The model under review builds one solid part; all positions refer to its coordinate system, in mm. Face numbers are marked on the shaded views. A direction names the side the tool comes from. Round coordinates to 2 decimals unless told otherwise and drop trailing zeros. Write each loop counter-clockwise with the first axis right and the second up, starting at its lowest first coordinate (ties: lowest second). Pieces come first, ordered by that corner, then holes. Notation, with made-up numbers: (55.25, 57.5) - (62.25, 57.5) arc R18 cw to (62.25, 91.5) - close; hole circle Ø7 at (-37, 60.25). An arc over 180 degrees is marked (long way). Return JSON: item names as keys, results as strings.
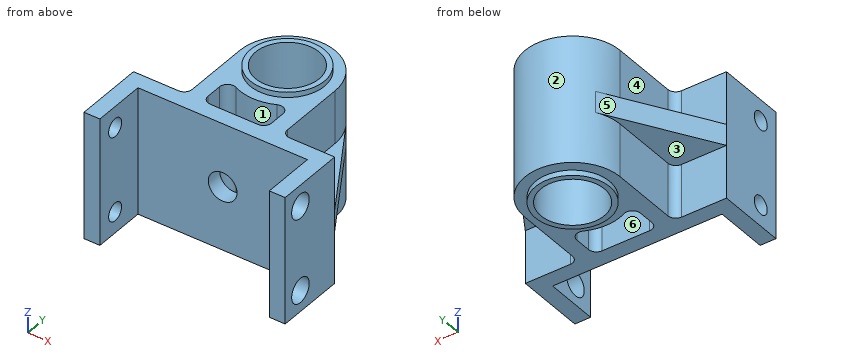
from build123d import *

# Parameters (mm, degrees)
F0_R           = 4.7625
F1_DEPTH       = 19.05
F2_R           = 1.8288
F3_DEPTH       = 2.38125
F4_R           = 1.35255
F5_DEPTH       = 2.38125
F8_DEPTH       = 1.5875
F9_R           = 5.55625
F9_R_2         = 4.7625
F11_DEPTH      = 0.79375
F11_DEPTH_BACK = 19.84375
F12_R          = 1.7272
F13_DEPTH      = 10.0554862042
F15_DEPTH      = 19.05
F16_R          = 2.15265
F17_DEPTH      = 2.38125
F18_R          = 1.190625


with BuildPart() as f1:
    # F0 (on Top) → F1 (new body)
    with BuildSketch(Plane.XY):
        with BuildLine():
            Line((7.14375, -11.1125), (7.14375, 0))
            ThreePointArc((7.14375, 0), (0, 7.14375), (-7.14375, 0))
            Line((-7.14375, 0), (-7.14375, -11.1125))
            Line((-7.14375, -11.1125), (-15.08125, -11.1125))
            Line((-15.08125, -11.1125), (-15.08125, -21.43125))
            Line((-15.08125, -21.43125), (-12.7, -21.43125))
            Line((-12.7, -21.43125), (-12.7, -13.49375))
            Line((-12.7, -13.49375), (12.7, -13.49375))
            Line((12.7, -13.49375), (12.7, -21.43125))
            Line((12.7, -21.43125), (15.08125, -21.43125))
            Line((15.08125, -21.43125), (15.08125, -11.1125))
            Line((15.08125, -11.1125), (7.14375, -11.1125))
        make_face()
        Circle(F0_R, mode=Mode.SUBTRACT)
    extrude(amount=F1_DEPTH)

    # F2 (on face) → F3 (cut, through all)
    with BuildSketch(Plane.YZ.offset(15.08125)):
        with Locations((-18.25625, 15.875)):
            Circle(F2_R)
        with Locations((-18.25625, 3.175)):
            Circle(F2_R)
    extrude(amount=-F3_DEPTH, mode=Mode.SUBTRACT)

    # F4 (on face) → F5 (cut, through all)
    with BuildSketch(Plane(origin=(-15.08125, 0, 0), x_dir=(0, -1, 0), z_dir=(-1, 0, 0))):
        with Locations((18.25625, 3.175)):
            Circle(F4_R)
        with Locations((18.25625, 15.875)):
            Circle(F4_R)
    extrude(amount=-F5_DEPTH, mode=Mode.SUBTRACT)

    # F7 (on offset) → F8 (join, symmetric)
    with BuildSketch(Plane(origin=(0, 0, 9.525), x_dir=(1, 0, 0), z_dir=(0, 0, -1))):
        with BuildLine():
            Line((-15.08125, 11.1125), (-6.1105859798, -3.7005274011))
            ThreePointArc((-6.1105859798, -3.7005274011), (-6.8806127146, -1.9210238767), (-7.14375, 0))
            Line((-7.14375, 0), (-7.14375, 11.1125))
            Line((-7.14375, 11.1125), (-15.08125, 11.1125))
        make_face()
        with BuildLine():
            ThreePointArc((7.14375, 0), (6.8806127146, -1.9210238767), (6.1105859798, -3.7005274011))
            Line((6.1105859798, -3.7005274011), (15.08125, 11.1125))
            Line((15.08125, 11.1125), (7.14375, 11.1125))
            Line((7.14375, 11.1125), (7.14375, 0))
        make_face()
    extrude(amount=F8_DEPTH, both=True)

    # F9 (on face) → F11 (join, two sides)
    with BuildSketch(Plane(origin=(0, 0, 0), x_dir=(1, 0, 0), z_dir=(0, 0, -1))) as f11_sk:
        Circle(F9_R)
        Circle(F9_R_2, mode=Mode.SUBTRACT)
    extrude(amount=F11_DEPTH)
    extrude(f11_sk.sketch, amount=-F11_DEPTH_BACK)

    # F12 (on face) → F13 (cut, up to face)
    with BuildSketch(Plane.XZ.offset(13.49375)):
        with Locations((0, 9.525)):
            Circle(F12_R)
    extrude(amount=-F13_DEPTH, mode=Mode.SUBTRACT)

    # F14 (on face) → F15 (cut, through all)
    with BuildSketch(Plane.XY.offset(19.05)):
        with BuildLine():
            Line((-4.7625, -5.3246368714), (-4.7625, -11.1125))
            Line((-4.7625, -11.1125), (4.7625, -11.1125))
            Line((4.7625, -11.1125), (4.7625, -5.3246368714))
            ThreePointArc((4.7625, -5.3246368714), (0, -7.14375), (-4.7625, -5.3246368714))
        make_face()
    extrude(amount=-F15_DEPTH, mode=Mode.SUBTRACT)

    # F16 (on face) → F17 (cut, through all)
    with BuildSketch(Plane.XZ.offset(13.49375)):
        with Locations((0, 9.525)):
            Circle(F16_R)
    extrude(amount=-F17_DEPTH, mode=Mode.SUBTRACT)

    # F18
    f18_edges = [f1.edges().sort_by_distance(p)[0] for p in [
        (7.14375, -11.1125, 15.08125),
        (7.14375, -11.1125, 3.96875),
        (-7.14375, -11.1125, 15.08125),
        (-7.14375, -11.1125, 3.96875),
        (-4.7625, -11.1125, 9.525),
        (4.7625, -11.1125, 9.525),
        (4.7625, -5.324637, 9.525),
        (-4.7625, -5.324637, 9.525),
    ]]
    fillet(f18_edges, radius=F18_R)


solid = f1.part
(1) Add section D-D (y = 2.5). Write out the cut boundary in (x, z).
Filled in:
{"outline": "(-6.84, 7.94) - (-6.69, 7.94) - (-6.69, 0) - (-4.96, 0) - (-4.96, -0.79) - (-4.05, -0.79) - (-4.05, 19.84) - (-4.96, 19.84) - (-4.96, 19.05) - (-6.69, 19.05) - (-6.69, 11.11) - (-6.84, 11.11) - close; (4.05, -0.79) - (4.96, -0.79) - (4.96, 0) - (6.69, 0) - (6.69, 7.94) - (6.84, 7.94) - (6.84, 11.11) - (6.69, 11.11) - (6.69, 19.05) - (4.96, 19.05) - (4.96, 19.84) - (4.05, 19.84) - close"}
(2) Add section C-C (z = 12.5). Write out the cut boundary in (x, y) (1 decimal), plus the area to 3 significant figures.
Filled in:
{"outline": "(-15.1, -21.4) - (-12.7, -21.4) - (-12.7, -13.5) - (12.7, -13.5) - (12.7, -21.4) - (15.1, -21.4) - (15.1, -11.1) - (8.3, -11.1) arc R1.2 cw to (7.1, -9.9) - (7.1, 0) arc R7.1 ccw to (-7.1, 0) - (-7.1, -9.9) arc R1.2 cw to (-8.3, -11.1) - (-15.1, -11.1) - close; hole (-4.8, -9.9) arc R1.2 ccw to (-3.6, -11.1) - (3.6, -11.1) arc R1.2 ccw to (4.8, -9.9) - (4.8, -7.5) arc R1.2 ccw to (3.1, -6.5) arc R7.1 cw to (-3.1, -6.5) arc R1.2 ccw to (-4.8, -7.5) - close; hole circle Ø9.5 at (0, 0)", "area": "237 mm2"}
(3) Wall thickness on line 1 (X direction, y = -8, z = 18.5); line 2 (X direction, y = -20, z = 1.25); line 3 (Y direction, x = 0, z = 12): over which ranges is each line inside the solid? List them lowest first.
Filled in:
{"line 1": "x = -7.14 to -4.76, 4.76 to 7.14", "line 2": "x = -15.08 to -12.7, 12.7 to 15.08", "line 3": "y = -13.49 to -11.11, -7.14 to -4.76, 4.76 to 7.14"}
(4) Clearance check with flat-ended pins moving along their axes: pin 1 Ø1 at (x, y) = (6, -5.5) entering from -Z; pin 2 Ø1.2 at (y, z) = (-9, 10.5) entering from -X; pin 3 Ø4 at (x, z) = (3.5, 8) entering from -Y. State where each tip first meets the part, or that it passes through.
Filled in:
{"pin 1": "stops at z = 0", "pin 2": "stops at x = -14.17", "pin 3": "stops at y = -13.49"}
(5) Add section A-A (x = 0). Write out the cut boundary in (y, z).
Filled in:
{"outline": "(-13.49, 0) - (-11.11, 0) - (-11.11, 7.37) - (-13.49, 7.37) - close; (-13.49, 11.68) - (-11.11, 11.68) - (-11.11, 19.05) - (-13.49, 19.05) - close; (-7.14, 0) - (-5.56, 0) - (-5.56, -0.79) - (-4.76, -0.79) - (-4.76, 7.8) - (-7.14, 7.8) - close; (-7.14, 11.25) - (-4.76, 11.25) - (-4.76, 19.84) - (-5.56, 19.84) - (-5.56, 19.05) - (-7.14, 19.05) - close; (4.76, -0.79) - (5.56, -0.79) - (5.56, 0) - (7.14, 0) - (7.14, 19.05) - (5.56, 19.05) - (5.56, 19.84) - (4.76, 19.84) - close"}
(6) For the marked faces 1, 2 and 3, list the 3-axis set-ups (+Z, -Z, +X, -X, +Y, -Y) from which the entire face can be reached by the end or side of a thin tool; tool diameter is ignored.
Filled in:
{"face 1": "+Z, -Z", "face 2": "+Y", "face 3": "-Z, -X, +Y"}
(7) Mouldability with a two-part tool opening along Y and no side actions: class the marked faces 4, 5 and 6 as released by +Y, released by -Y, zero draft, split by the parting line, or undercut.
Filled in:
{"face 4": "zero draft", "face 5": "released by +Y", "face 6": "undercut"}
(8) Add section B-B (z = 15.5). Give the number of separate pieces and of enclosed holes in the cut face, plus the area to 3 significant figures.
Filled in:
{"separate pieces": "3", "enclosed holes": "2", "area": "223 mm2"}
